from build123d import *

# Parameters (mm, degrees)
SKETCH3_R          = 1.6
CUT_EXTRUDE1_DEPTH = 95.098950047
CIRPATTERN1_COUNT  = 12


with BuildPart() as part:
    # Sketch1 → Revolve1 (revolve)
    with BuildSketch(Plane.XY, mode=Mode.PRIVATE) as revolve1_sk:
        with BuildLine():
            Line((-66.5, 9.851956719), (-66.5, 9.965))
            Line((-66.5, 9.965), (-60, 9.965))
            Line((-60, 9.965), (-60, 6.785))
            Line((-60, 6.785), (-66.5, 6.785))
            Line((-66.5, 6.785), (-66.5, 7.218043281))
            ThreePointArc((-66.5, 7.218043281), (-66, 8.535), (-66.5, 9.851956719))
        make_face()
    revolve(revolve1_sk.sketch.rotate(Axis((0, -200069.047495165, 0), (0, 1, 0)), 270), axis=Axis((0, -200069.047495165, 0), (0, 1, 0)))

    # Sketch3 → Cut-Extrude1 (cut, through all)
    with BuildSketch(Plane(origin=(0, 9.965, 0), x_dir=(1, 0, 0), z_dir=(0, 1, 0))):
        with Locations(Location((0, 63, 0), (0, 0, 270))):
            Circle(SKETCH3_R)
    cut_extrude1 = extrude(amount=-CUT_EXTRUDE1_DEPTH, mode=Mode.SUBTRACT)

    # CirPattern1: Cut-Extrude1 ×12 about axis
    cirpattern1_axis = Axis((0, 0, 0), (0, 1, 0))
    for i in range(1, CIRPATTERN1_COUNT):
        add(cut_extrude1.rotate(cirpattern1_axis, i * 360 / CIRPATTERN1_COUNT), mode=Mode.SUBTRACT)


solid = part.part
Source: CAD feature listing. Evaluate the final solid. Frame: model axes, mm. Give positions to 0.01 mm unless a question says otherwise; leave off trailing zeros. Write each loop counter-clockwise with the first axis right and the second up, starting at its lowest first coordinate (ties: lowest second). Pieces come first, ordered by that corner, then holes. Notation, with made-up numbers: (9.25, 33) - (31.25, 33) arc R24 cw to (31.25, 53) - close; hole circle Ø5 at (71, 18.5). An arc over 180 degrees is marked (long way). Write item = value, one per line. Start each with the question number.
Q1. Cut plane A-A, the plane z = 0. Return loops of the section in (x, y) (3 decimals).
Q2. Material intervals for probe 1 along Z at (x, y) = (-31.5, 8.65); probe 2 along X at (y, z) = (8.7, -31.5); probe 3 along X at (y, z) = (7.9, 20), sorted ascending.
Q3. Cut plane B-B, the plane y = 8.25. Give the number of separate pieces and of enclosed holes in the cut face, then the cut area to 3 significant figures.
Q4. Draft query along Z for faces 1 (the cylindrical face through (-65.934, 7.005, 8.657)), 2 (the flat face through (-59.4, 6.785, -10.2)), 3 (the cylindrical face through (-52.973, 8.397, 31.292)). Return one class per face: +Z half, -Z half, draft (parallel to the pull), parting line (faces both ways), or undercut.
Q5. Pin query (flat end, axial travel): pin 1 Ø1.9 at (x, z) = (54.56, 31.5) entering from -Y; pin 2 Ø1.5 at (y, z) = (8, -25.5) entering from +X; pin 3 Ø1 at (x, y) = (-9, 9.5) entering from +Z; pin 4 Ø1 at (x, y) = (42, 8.5) entering from -Z. Return the tip coordinate at first contact, or that it passes through.
Computed values:
q1.outline = (-66.5, 6.785) - (-64.6, 6.785) - (-64.6, 9.965) - (-66.5, 9.965) - (-66.5, 9.852) arc R1.984 cw to (-66.5, 7.218) - close; (-61.4, 6.785) - (-60, 6.785) - (-60, 9.965) - (-61.4, 9.965) - close; (60, 6.785) - (61.4, 6.785) - (61.4, 9.965) - (60, 9.965) - close; (64.6, 6.785) - (66.5, 6.785) - (66.5, 7.218) arc R1.984 cw to (66.5, 9.852) - (66.5, 9.965) - (64.6, 9.965) - close
q2.probe_1 = -58 to -56.16, -52.96 to -51.07, 51.07 to 52.96, 56.16 to 58
q2.probe_2 = -58.01 to -56.16, -52.96 to -51.07, 51.07 to 52.96, 56.16 to 58.01
q2.probe_3 = -63.01 to -56.57, 56.57 to 63.01
q3.separate_pieces = 1
q3.enclosed_holes = 13
q3.area = 2,290 mm²
q4.face_1 = parting line
q4.face_2 = draft
q4.face_3 = undercut
q5.pin_1 = through
q5.pin_2 = 61.46
q5.pin_3 = 65.94
q5.pin_4 = -51.32
